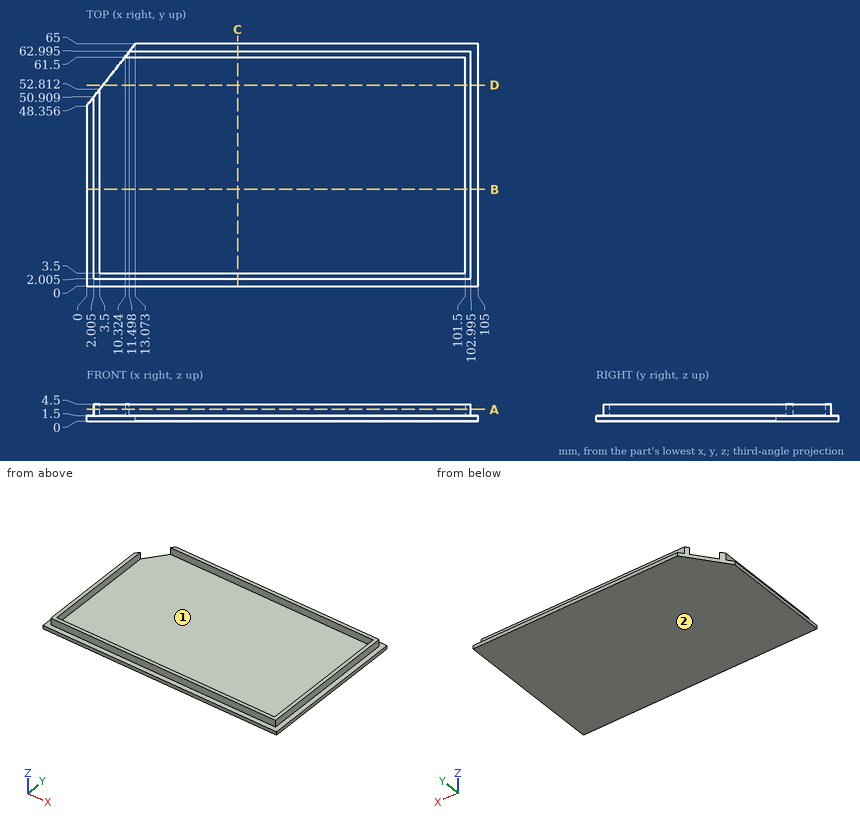
The figure shows three views and two pictorial views of one solid part (mm, origin at its lowest corner). Answer the questions. Coordinates: 2 decimals unless noted, no trailing zeros. Loops run counter-clockwise (first coordinate to the right, second up) from the corner with the lowest first, then second, coordinate; pieces in that order, holes last. Notation, with made-up numbers: (87.25, 65.5) -> (124.25, 65.5) arc R9 ccw to (124.25, 80.5) -> close; hole circle Ø1 at (-37, 80). An arc over 180 degrees is marked (long way). Write item = value, one per line. Start each with the question number.
1) Straight lines are drawn through the part: line 1 (X direction, y = 46, z = 2.9) (1 decimal); line 2 (Y direction, x = 12, z = 4.15) (1 decimal); line 3 (Z direction, x = 84, y = 29). For each, find the intervals that lie inside material, in ascending order. Write a range as from..to.
2) A cutting plane is placed at C-C (x = 40.5). Give the vertices of the cut face in (y, z) (1 decimal).
3) A cutting plane is placed at D-D (y = 54). Give the vertices of the cut face in (x, z) (1 decimal).
4) The mould has two halves that part along X. Classify the marked faces 1 and 2: released by +X, released by -X, zero draft, split by the parting line, or undercut.
5) A cutting plane is placed at A-A (z = 3.15). Give the vertices of the cut face in (x, y) (1 decimal).
6) A cutting plane is placed at B-B (y = 26). Give the vertices of the cut face in (x, z) (1 decimal).
7) Given pin 1 Ø1.5 at (x, z) = (28, 3.5) entering from -Y (3 decimals); pin 2 Ø0.9 at (y, z) = (35, 3.5) entering from -X (3 decimals); pin 3 Ø1.5 at (y, z) = (31.5, 2.5) entering from +X (3 decimals), each flat-ended and moving along its own axis, determine where each tip first touches the part or whether it passes through.
Responses:
q1.line_1 = 2..3.5, 101.5..103
q1.line_2 = 2..3.5, 61.5..63
q1.line_3 = 0..1.5
q2.outline = (0, 0) -> (65, 0) -> (65, 1.5) -> (63, 1.5) -> (63, 4.5) -> (61.5, 4.5) -> (61.5, 1.5) -> (3.5, 1.5) -> (3.5, 4.5) -> (2, 4.5) -> (2, 1.5) -> (0, 1.5) -> close
q3.outline = (4.4, 0) -> (105, 0) -> (105, 1.5) -> (103, 1.5) -> (103, 4.5) -> (101.5, 4.5) -> (101.5, 1.5) -> (4.4, 1.5) -> close
q4.face_1 = undercut
q4.face_2 = zero draft
q5.outline = (2, 2) -> (103, 2) -> (103, 63) -> (11.5, 63) -> (10.3, 61.5) -> (101.5, 61.5) -> (101.5, 3.5) -> (3.5, 3.5) -> (3.5, 52.8) -> (2, 50.9) -> close
q6.outline = (0, 0) -> (105, 0) -> (105, 1.5) -> (103, 1.5) -> (103, 4.5) -> (101.5, 4.5) -> (101.5, 1.5) -> (3.5, 1.5) -> (3.5, 4.5) -> (2, 4.5) -> (2, 1.5) -> (0, 1.5) -> close
q7.pin_1 = 2.005
q7.pin_2 = 2.005
q7.pin_3 = 102.995
